Input: part model. Units: mm. Frame: model coordinates. A direction names the side the tool comes from. Round coordinates to 2 decimals unless told otherwise and drop trailing zeros. Order: outer loops, then holes, each group sorted by start corner. A loop starts at its lowest first (then second) coordinate and runs counter-clockwise, first axis right, second up. Notation, with made-up numbers: (7, 12.5) -> (27, 12.5) arc R23 cw to (27, 33.5) -> close; hole circle Ø11 at (64.25, 68.5). An arc over 180 degrees is marked (long way). Answer as CSV lines item,"result". Start each with the question number.
1) Section query B-B, the plane y = 50.5. Output: boundary loops of the cut face in (x, z).
2) Section query C-C, the plane x = -27.5. Output: boundary loops of the cut face in (y, z), and give its area (3 significant figures).
3) Line query: L1, parallel to X at y = 22.5, z = 2.25; L2, parallel to X at y = 37, z = 5; L3, parallel to Y at x = 15, z = 5.65. Output: solid intervals per line, ascending.
4) Access query for faces 1 (the face through (-70, 67, 2)), 2 (the face through (11.1, -16.14, 3.55)), 3 (the face through (-55.95, -20.94, 2.07)). Directions: +Z, -Z, +X, -X, +Y, -Y. A direction counts if a zero-diameter tool reaches every point of the face in a straight line with its end or side. Return the directions, or none.
5) First-contact query: P1, Ø3.5, axis at x = -70, y = 65, coming from the +Z side. Flat tip, straight axial feed; report the tip coordinate or a pass-through.
6) Section query D-D, the plane z = 3.5. State how many separate pieces and enclosed holes the cut face has, and give its area (3 significant figures).
7) Mould query, pull axis Z, two halves, no side actions, for faces 4 (the face through (-71.846, 68.549, 4.535)), 5 (the face through (-70, 26, 0)), 6 (the face through (13, -20, 2)), 7 (the face through (1.075, -20.944, 2.114)). Classes: +Z half, -Z half, draft (parallel to the pull), parting line (faces both ways), or undercut.
8) Section query A-A, the plane x = -6. Output: boundary loops of the cut face in (y, z).
Autodesk Fusion 360 part; units mm, degrees
sketch "Sketch1" plane through (0, 0, 0) normal (0, 0, 1) x (1, 0, 0)
  line L0 (19, -25) -> (-74, -25)
  line L1 (-75, -24) -> (-75, 69)
  line L2 (-74, 70) -> (19, 70)
  line L3 (20, 69) -> (20, -24)
  arc A0 (-74, 70) -> (-75, 69) centre (-74, 69) ccw
  arc A1 (20, 69) -> (19, 70) centre (19, 69) ccw
  arc A2 (-75, -24) -> (-74, -25) centre (-74, -24) ccw
  arc A3 (19, -25) -> (20, -24) centre (19, -24) ccw
  point P0 (20, -25)
  point P1 (-75, -25)
  point P2 (20, 70)
  dimension "d1" = 95
  dimension "d2" = 95
  dimension "d3" = 1
extrude "Extrude1" add sketch "Sketch1" along normal blind 7
sketch "Sketch2" plane through (0, 0, 7) normal (0, 0, 1) x (-1, 0, 0)
  arc A0 (75, 24) -> (74, 25) centre (74, 24) ccw
  line L0 (74, 25) -> (-19, 25)
  arc A1 (-19, 25) -> (-20, 24) centre (-19, 24) ccw
  line L1 (-20, 24) -> (-20, -69)
  arc A2 (-20, -69) -> (-19, -70) centre (-19, -69) ccw
  line L2 (-19, -70) -> (74, -70)
  arc A3 (74, -70) -> (75, -69) centre (74, -69) ccw
  line L3 (75, -69) -> (75, 24)
  line L4 (64, -62) -> (-9, -62)
  line L5 (-12, -59) -> (-12, 14)
  line L6 (-9, 17) -> (64, 17)
  line L7 (67, 14) -> (67, -59)
  arc A4 (64, -62) -> (67, -59) centre (64, -59) ccw
  arc A5 (-12, -59) -> (-9, -62) centre (-9, -59) ccw
  arc A6 (-9, 17) -> (-12, 14) centre (-9, 14) ccw
  arc A7 (67, 14) -> (64, 17) centre (64, 14) ccw
  point P0 (67, -62)
  point P1 (-12, -62)
  point P2 (67, 17)
  dimension "d6" = 79
  dimension "d7" = 79
  dimension "d8" = 3
  dimension "d9" = 8
  dimension "d10" = 8
extrude "Extrude2" cut sketch "Sketch2" against normal blind 19 contours L4 L5 L6 L7 A4 A5 A6 A7
sketch "Sketch3" plane through (0, 0, 7) normal (0, 0, 1) x (-1, 0, 0)
  line L0 (67, 14) -> (67, -59)
  arc A0 (64, -62) -> (67, -59) centre (64, -59) ccw
  line L1 (64, -62) -> (-9, -62)
  arc A1 (-12, -59) -> (-9, -62) centre (-9, -59) ccw
  line L2 (-12, -59) -> (-12, 14)
  arc A2 (-9, 17) -> (-12, 14) centre (-9, 14) ccw
  line L3 (-9, 17) -> (64, 17)
  arc A3 (67, 14) -> (64, 17) centre (64, 14) ccw
  arc A4 (75, 24) -> (74, 25) centre (74, 24) ccw
  line L4 (74, 25) -> (-19, 25)
  arc A5 (-19, 25) -> (-20, 24) centre (-19, 24) ccw
  line L5 (-20, 24) -> (-20, -69)
  arc A6 (-20, -69) -> (-19, -70) centre (-19, -69) ccw
  line L6 (-19, -70) -> (74, -70)
  arc A7 (74, -70) -> (75, -69) centre (74, -69) ccw
  line L7 (75, -69) -> (75, 24)
  point P0 (27.5, 21)
  point P1 (71, -22.5)
  point P2 (-16, -22.5)
  point P3 (27.5, -66)
  dimension "d13" = 4
  dimension "d14" = 47.5
  dimension "d15" = 4
  dimension "d16" = 47.5
  dimension "d17" = 4
  dimension "d18" = 47.5
  dimension "d19" = 4
  dimension "d20" = 47.5
hole "Hole1" at (-27.5, 66, 7) at (16, 22.5, 7) at (-27.5, -21, 7) at (-71, 22.5, 7) direction (0, 0, -1) diameter 3 depth 25 tip angle 118
sketch "Sketch4" plane through (0, -25, 0) normal (0, -1, 0) x (1, 0, 0)
  line L0 (-74, 0) -> (19, 0)
  line L1 (19, 0) -> (19, 7)
  line L2 (19, 7) -> (-74, 7)
  line L3 (-74, 7) -> (-74, 0)
  line L4 (-75, 0) -> (-75, 7)
  point P0 (-27.5, 3.5)
  point P1 (-55.5, 3.5)
  point P2 (0.5, 3.5)
  dimension "d24" = 3.5
  dimension "d25" = 3.5
  dimension "d26" = 3.5
  dimension "d27" = 47.5
  dimension "d28" = 28
  dimension "d29" = 28
hole "Hole2" at (-55.5, -25, 3.5) at (0.5, -25, 3.5) direction (0, 1, 0) diameter 3 depth 124 tip angle 118
sketch "Sketch5" plane through (20, 0, 0) normal (1, 0, 0) x (0, 1, 0)
  line L0 (-24, 0) -> (69, 0)
  line L1 (69, 0) -> (69, 7)
  line L2 (69, 7) -> (-24, 7)
  line L3 (-24, 7) -> (-24, 0)
  line L4 (-25, 0) -> (-25, 7)
  point P0 (-5.5, 3.5)
  point P1 (22.5, 3.5)
  point P2 (50.5, 3.5)
  dimension "d33" = 3.5
  dimension "d34" = 3.5
  dimension "d35" = 3.5
  dimension "d36" = 47.5
  dimension "d37" = 28
  dimension "d38" = 28
hole "Hole3" at (20, -5.5, 3.5) at (20, 50.5, 3.5) direction (-1, 0, 0) diameter 3 depth 124 tip angle 118
sketch "Sketch6" plane through (0, 0, 7) normal (0, 0, 1) x (-1, 0, 0)
  circle A0 centre (27.5, 21) radius 1.5
  circle A1 centre (27.5, -66) radius 1.5
  circle A2 centre (-16, -22.5) radius 1.5
  circle A3 centre (71, -22.5) radius 1.5
  line L0 (67, 14) -> (67, -59)
  arc A4 (64, -62) -> (67, -59) centre (64, -59) ccw
  line L1 (64, -62) -> (-9, -62)
  arc A5 (-12, -59) -> (-9, -62) centre (-9, -59) ccw
  line L2 (-12, -59) -> (-12, 14)
  arc A6 (-9, 17) -> (-12, 14) centre (-9, 14) ccw
  line L3 (-9, 17) -> (64, 17)
  arc A7 (67, 14) -> (64, 17) centre (64, 14) ccw
  arc A8 (75, 24) -> (74, 25) centre (74, 24) ccw
  line L4 (74, 25) -> (-19, 25)
  arc A9 (-19, 25) -> (-20, 24) centre (-19, 24) ccw
  line L5 (-20, 24) -> (-20, -69)
  arc A10 (-20, -69) -> (-19, -70) centre (-19, -69) ccw
  line L6 (-19, -70) -> (74, -70)
  arc A11 (74, -70) -> (75, -69) centre (74, -69) ccw
  line L7 (75, -69) -> (75, 24)
  point P0 (70, 20)
  point P1 (-15, 20)
  point P2 (70, -65)
  point P3 (-15, -65)
  dimension "d42" = 5
  dimension "d43" = 5
  dimension "d44" = 5
  dimension "d45" = 5
  dimension "d46" = 5
  dimension "d47" = 5
  dimension "d48" = 5
  dimension "d49" = 5
hole "Hole4" at (15, 65, 7) at (-70, 65, 7) at (-70, -20, 7) at (15, -20, 7) direction (0, 0, -1) diameter 3 depth 10 tip angle 118
sketch "Sketch7" plane through (0, 0, 7) normal (0, 0, 1) x (-1, 0, 0)
  circle A0 centre (70, 20) radius 1.5
  circle A1 centre (-15, -65) radius 1.5
  circle A2 centre (70, -65) radius 1.5
  circle A3 centre (-15, 20) radius 1.5
  circle A4 centre (27.5, 21) radius 1.5
  circle A5 centre (27.5, -66) radius 1.5
  circle A6 centre (-16, -22.5) radius 1.5
  circle A7 centre (71, -22.5) radius 1.5
  line L0 (67, 14) -> (67, -59)
  arc A8 (64, -62) -> (67, -59) centre (64, -59) ccw
  line L1 (64, -62) -> (-9, -62)
  arc A9 (-12, -59) -> (-9, -62) centre (-9, -59) ccw
  line L2 (-12, -59) -> (-12, 14)
  arc A10 (-9, 17) -> (-12, 14) centre (-9, 14) ccw
  line L3 (-9, 17) -> (64, 17)
  arc A11 (67, 14) -> (64, 17) centre (64, 14) ccw
  arc A12 (75, 24) -> (74, 25) centre (74, 24) ccw
  line L4 (74, 25) -> (-19, 25)
  arc A13 (-19, 25) -> (-20, 24) centre (-19, 24) ccw
  line L5 (-20, 24) -> (-20, -69)
  arc A14 (-20, -69) -> (-19, -70) centre (-19, -69) ccw
  line L6 (-19, -70) -> (74, -70)
  arc A15 (74, -70) -> (75, -69) centre (74, -69) ccw
  line L7 (75, -69) -> (75, 24)
  circle A16 centre (70, -65) radius 4
  circle A17 centre (-15, -65) radius 4
  circle A18 centre (70, 20) radius 4
  circle A19 centre (-15, 20) radius 4
  dimension "d53" = 8
  dimension "d54" = 8
  dimension "d55" = 8
  dimension "d56" = 8
extrude "Extrude3" cut sketch "Sketch7" against normal blind 5 contours A16 | A17 | A18 | A19
Findings:
1,outline,"(-75, 0) -> (-67, 0) -> (-67, 2) -> (-75, 2) -> close; (-75, 5) -> (-67, 5) -> (-67, 7) -> (-75, 7) -> close; (12, 0) -> (20, 0) -> (20, 2) -> (12, 2) -> close; (12, 5) -> (20, 5) -> (20, 7) -> (12, 7) -> close"
2,outline,"(-25, 0) -> (-22.5, 0) -> (-22.5, 7) -> (-25, 7) -> close; (-19.5, 0) -> (-17, 0) -> (-17, 7) -> (-19.5, 7) -> close; (62, 0) -> (64.5, 0) -> (64.5, 7) -> (62, 7) -> close; (67.5, 0) -> (70, 0) -> (70, 7) -> (67.5, 7) -> close"
2,area,"70.0 mm^2"
3,L1,"x = -75 to -72.5, -69.5 to -67, 12 to 14.5, 17.5 to 20"
3,L2,"x = -75 to -67, 12 to 20"
3,L3,"y = -25 to -24, -16 to 21.38, 23.62 to 61, 69 to 70"
4,face 1,"+Z"
4,face 2,"+Z, -Z"
4,face 3,"+Y, -Y"
5,P1,"stops at z = 2"
6,separate pieces,"8"
6,enclosed holes,"8"
6,area,"2,370 mm^2"
7,face 4,"draft"
7,face 5,"-Z half"
7,face 6,"+Z half"
7,face 7,"undercut"
8,outline,"(-25, 0) -> (-17, 0) -> (-17, 7) -> (-25, 7) -> close; (62, 0) -> (70, 0) -> (70, 7) -> (62, 7) -> close"
